Geometry: see drawing. Coordinates: mm, zero at the bounding-box minimum. A direction names the side the tool comes from. Coordinates: 2 decimals unless noted, no trailing zeros. Order: outer loops, then holes, each group sorted by start corner. A loop starts at its lowest first (then second) coordinate and runs counter-clockwise, first axis right, second up. Notation, with made-up numbers: M -4.75,21.25 L 23.25,21.25 A19 cw 23.25,27.25 Z; hole C 26.5,77.25 d2. An arc over 180 degrees is marked long. One line per item, written item: value.
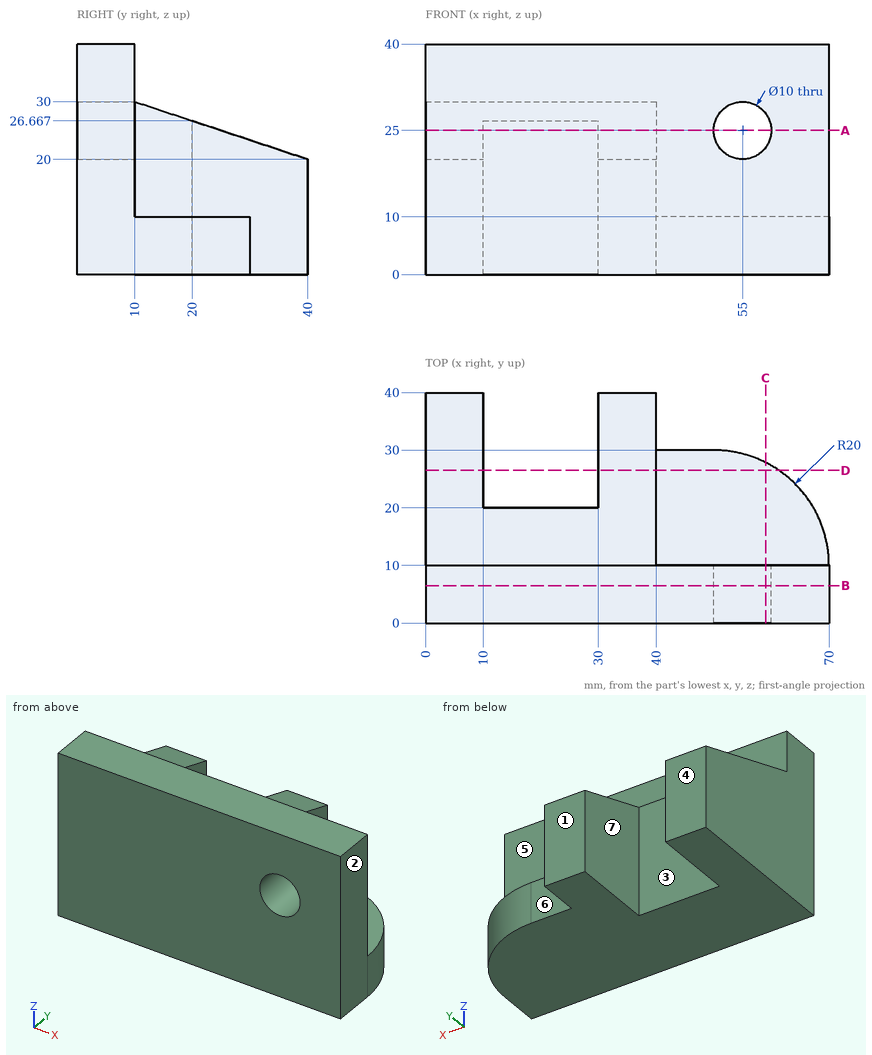
(1) Cut plane B-B on y = 6.5. Output: boundary loops of the cut face in (x, z).
Data:
outline: M 0,0 L 70,0 L 70,40 L 0,40 Z; hole C 55,25 d10
(2) First-contact query: pin 1 (3 mm diameter, centred on x = 44.5, z = 3, fed in from +Y); pin 2 (13 mm diameter, centred on x = 55, z = 25, fed in from +Y); pin 3 (6 mm diameter, centred on y = 35, z = 7.5, fed in from +X). Flat tips, straight axial feed; report the tip coordinate or a pass-through.
Data:
pin 1: stops at y = 30
pin 2: stops at y = 10
pin 3: stops at x = 40
(3) Cut plane A-A on z = 25. Output: boundary loops of the cut face in (x, y), plus the area to 3 significant figures.
Data:
outline: M 0,0 L 50,0 L 50,10 L 40,10 L 40,25 L 30,25 L 30,20 L 10,20 L 10,25 L 0,25 Z; M 60,0 L 70,0 L 70,10 L 60,10 Z
area: 1,100 mm2
(4) Draft query along X for the marked faces 1, 2 and 3. Return one class per face: released by +X, released by -X, zero draft, split by the parting line, or undercut.
Data:
face 1: zero draft
face 2: released by +X
face 3: undercut
(5) Ray query, line 1 (Z direction, x = 55, y = 4); line 2 (X direction, y = 26, z = 23); line 3 (X direction, y = 6.25, z = 25). Return the intervals inside material, ascending. Write a range as from..to.
Data:
line 1: z = 0..20, 30..40
line 2: x = 0..10, 30..40
line 3: x = 0..50, 60..70
(6) Access query for the marked faces 4, 5, 6 and 7. Directions: +Z, -Z, +X, -X, +Y, -Y. A direction counts if a zero-diameter tool reaches every point of the face in a straight line with its end or side. Return the directions, or none.
Data:
face 4: +Z, -Z, +X, -X, +Y
face 5: +Z, +X, +Y
face 6: +Z, -Z, +X, +Y
face 7: +Z, -Z, +Y
(7) Cut plane D-D on y = 26.5. Output: boundary loops of the cut face in (x, z), plus the area to 3 significant figures.
Data:
outline: M 0,0 L 10,0 L 10,24.5 L 0,24.5 Z; M 30,0 L 61.3,0 L 61.3,10 L 40,10 L 40,24.5 L 30,24.5 Z
area: 703 mm2
(8) Cut plane C-C on x = 59. Output: boundary loops of the cut face in (y, z).
Data:
outline: M 0,0 L 27.86,0 L 27.86,10 L 10,10 L 10,22 L 0,22 Z; M 0,28 L 10,28 L 10,40 L 0,40 Z
